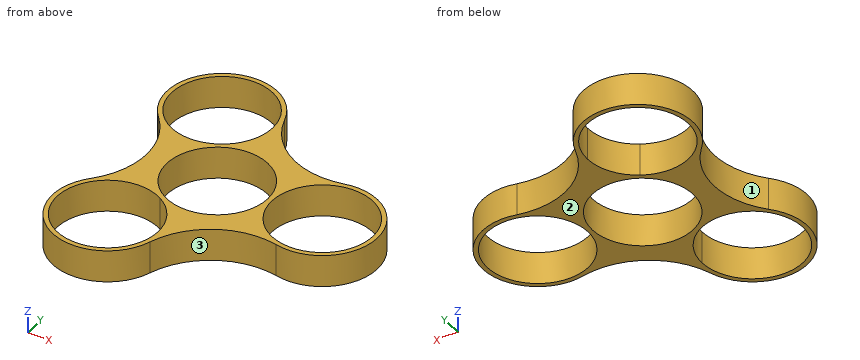
from build123d import *

# Parameters (mm, degrees)
F0_R     = 11
F1_DEPTH = 7


with BuildPart() as f1:
    # F0 (on Top) → F1 (new body)
    with BuildSketch(Plane.XY):
        with BuildLine():
            ThreePointArc((11.5, 3.427827), (11.874342, 1.732051), (12, 0))
            ThreePointArc((12, 0), (11.874342, -1.732051), (11.5, -3.427827))
            ThreePointArc((11.5, -3.427827), (14.754622, -8.718586), (20.218586, -11.673206))
            ThreePointArc((20.218586, -11.673206), (35, 0), (20.218586, 11.673206))
            ThreePointArc((20.218586, 11.673206), (14.754622, 8.718586), (11.5, 3.427827))
        make_face()
        with BuildLine():
            ThreePointArc((34, 0), (23, -11), (12, 0))
            ThreePointArc((12, 0), (23, 11), (34, 0))
        make_face(mode=Mode.SUBTRACT)
        with BuildLine():
            ThreePointArc((-2.781414, 11.673206), (6, 10.392305), (11.5, 3.427827))
            ThreePointArc((11.5, 3.427827), (14.754622, 8.718586), (20.218586, 11.673206))
            ThreePointArc((20.218586, 11.673206), (7.853112, 13.601989), (0, 23.346412))
            ThreePointArc((0, 23.346412), (0.173206, 17.13717), (-2.781414, 11.673206))
        make_face()
        with BuildLine():
            ThreePointArc((20.218586, -11.673206), (14.754622, -8.718586), (11.5, -3.427827))
            ThreePointArc((11.5, -3.427827), (6, -10.392305), (-2.781414, -11.673206))
            ThreePointArc((-2.781414, -11.673206), (0.173206, -17.13717), (0, -23.346412))
            ThreePointArc((0, -23.346412), (7.853112, -13.601989), (20.218586, -11.673206))
        make_face()
        with BuildLine():
            ThreePointArc((-6, 10.392305), (-4.437171, 11.149507), (-2.781414, 11.673206))
            ThreePointArc((-2.781414, 11.673206), (0.173206, 17.13717), (0, 23.346412))
            ThreePointArc((0, 23.346412), (-17.5, 30.310889), (-20.218586, 11.673206))
            ThreePointArc((-20.218586, 11.673206), (-14.927827, 8.418584), (-8.718586, 8.245378))
            ThreePointArc((-8.718586, 8.245378), (-7.437171, 9.417457), (-6, 10.392305))
        make_face()
        with BuildLine():
            ThreePointArc((-0.5, 19.918584), (-1.973721, 14.418584), (-6, 10.392305))
            ThreePointArc((-6, 10.392305), (-21.026279, 25.418584), (-0.5, 19.918584))
        make_face(mode=Mode.SUBTRACT)
        with BuildLine():
            ThreePointArc((0, -23.346412), (0.173206, -17.13717), (-2.781414, -11.673206))
            ThreePointArc((-2.781414, -11.673206), (-4.437171, -11.149507), (-6, -10.392305))
            ThreePointArc((-6, -10.392305), (-7.437171, -9.417457), (-8.718586, -8.245378))
            ThreePointArc((-8.718586, -8.245378), (-14.927827, -8.418584), (-20.218586, -11.673206))
            ThreePointArc((-20.218586, -11.673206), (-17.5, -30.310889), (0, -23.346412))
        make_face()
        with BuildLine():
            ThreePointArc((-0.5, -19.918584), (-21.02628, -25.418584), (-6, -10.392305))
            ThreePointArc((-6, -10.392305), (-1.97372, -14.418584), (-0.5, -19.918584))
        make_face(mode=Mode.SUBTRACT)
        with BuildLine():
            ThreePointArc((-8.718586, -8.245378), (-12, 0), (-8.718586, 8.245378))
            ThreePointArc((-8.718586, 8.245378), (-14.927827, 8.418584), (-20.218586, 11.673206))
            ThreePointArc((-20.218586, 11.673206), (-15.706224, 0), (-20.218586, -11.673206))
            ThreePointArc((-20.218586, -11.673206), (-14.927827, -8.418584), (-8.718586, -8.245378))
        make_face()
        with BuildLine():
            ThreePointArc((11.5, -3.427827), (11.874342, -1.732051), (12, 0))
            ThreePointArc((12, 0), (11.874342, 1.732051), (11.5, 3.427827))
            ThreePointArc((11.5, 3.427827), (6, 10.392305), (-2.781414, 11.673206))
            ThreePointArc((-2.781414, 11.673206), (-4.437171, 11.149507), (-6, 10.392305))
            ThreePointArc((-6, 10.392305), (-7.437171, 9.417457), (-8.718586, 8.245378))
            ThreePointArc((-8.718586, 8.245378), (-12, 0), (-8.718586, -8.245378))
            ThreePointArc((-8.718586, -8.245378), (-7.437171, -9.417457), (-6, -10.392305))
            ThreePointArc((-6, -10.392305), (-4.437171, -11.149507), (-2.781414, -11.673206))
            ThreePointArc((-2.781414, -11.673206), (6, -10.392305), (11.5, -3.427827))
        make_face()
        Circle(F0_R, mode=Mode.SUBTRACT)
    extrude(amount=F1_DEPTH)


solid = f1.part
The listing builds one solid part. Answer for the finished solid, in the listing's coordinates (mm). Face numbers are marked on the shaded views. Round coordinates to 2 decimals unless told otherwise and drop trailing zeros. Write each loop counter-clockwise with the first axis right and the second up, starting at its lowest first coordinate (ties: lowest second). Pieces come first, ordered by that corner, then holes. Notation, with made-up numbers: (17, 14.25) - (38, 14.25) arc R30 ccw to (38, 39.25) - close; hole circle Ø1 at (-30, 17). An arc over 180 degrees is marked (long way). Use one line per item in the form item = value. Start each with the question number.
Item 1: Flat-ended cylindrical pins translate along their axes: pin 1 Ø2 at (x, z) = (27, 3.5) entering from +Y; pin 2 Ø1.5 at (x, z) = (2.5, 1) entering from -Y; pin 3 Ø2 at (y, z) = (20, 2.5) entering from +X; pin 4 Ø10 at (x, y) = (8, -7.5) entering from +Z. Find the tip coordinate at first contact, or state that the pin passes through.
Item 2: A cutting plane is placed at D-D (x = -1.5). Write down the section's boundary in (y, z), plus the area to 3 significant figures.
Item 3: A cutting plane is placed at B-B (y = 0). Write down the section's boundary in (x, z), plus the area to 3 significant figures.
Item 4: A cutting plane is placed at A-A (z = 5). Write down the section's boundary in (x, y), plus the area to 3 significant figures.
Item 5: Find the intervals of material crossed by line 1 (Y direction, x = -11.5, z = 1.75); line 2 (Y direction, x = -19.5, z = 2.75); line 3 (Y direction, x = -5.5, z = 3.5), in increasing order. Write a range as [from, to].
Item 6: A cutting plane is placed at C-C (x = 23). Write down the section's boundary in (y, z).
Item 7: Determine the mould class of the marked faces 1, 2 and 3 for opening direction X: +X half, -X half, draft (parallel to the pull), parting line (faces both ways), or undercut.
The answers:
q1.pin_1 = 11.62
q1.pin_2 = -19.54
q1.pin_3 = 2.09
q1.pin_4 = 7
q2.outline = (-26.55, 0) - (-24.5, 0) - (-24.5, 7) - (-26.55, 7) - close; (-15.34, 0) - (-10.9, 0) - (-10.9, 7) - (-15.34, 7) - close; (10.9, 0) - (15.34, 0) - (15.34, 7) - (10.9, 7) - close; (24.5, 0) - (26.55, 0) - (26.55, 7) - (24.5, 7) - close
q2.area = 90.9 mm^2
q3.outline = (-15.71, 0) - (-11, 0) - (-11, 7) - (-15.71, 7) - close; (11, 0) - (12, 0) - (12, 7) - (11, 7) - close; (34, 0) - (35, 0) - (35, 7) - (34, 7) - close
q3.area = 46.9 mm^2
q4.outline = (-20.22, -11.67) arc R12 ccw (long way) to (0, -23.35) arc R17.36 cw to (20.22, -11.67) arc R12 ccw (long way) to (20.22, 11.67) arc R17.36 cw to (0, 23.35) arc R12 ccw (long way) to (-20.22, 11.67) arc R17.36 cw to start; hole circle Ø22 at (0, 0); hole (-6, -10.39) arc R11 ccw (long way) to (-0.5, -19.92) arc R11 ccw to start; hole (-6, 10.39) arc R11 ccw to (-0.5, 19.92) arc R11 ccw (long way) to start; hole circle Ø22 at (23, 0)
q4.area = 556 mm^2
q5.line_1 = [-31.92, -30.92], [-8.92, 8.92], [30.92, 31.92]
q5.line_2 = [-28.86, -27.47], [-12.37, -10.83], [10.83, 12.37], [27.47, 28.86]
q5.line_3 = [-30.31, -29.14], [-10.7, -9.53], [9.53, 10.7], [29.14, 30.31]
q6.outline = (-12, 0) - (-11, 0) - (-11, 7) - (-12, 7) - close; (11, 0) - (12, 0) - (12, 7) - (11, 7) - close
q7.face_1 = -X half
q7.face_2 = draft
q7.face_3 = undercut
